The model under review builds one solid part; all positions refer to its coordinate system, in mm. A direction names the side the tool comes from. Round coordinates to 2 decimals unless told otherwise and drop trailing zeros. Loops run counter-clockwise (first coordinate to the right, second up) from the corner with the lowest first, then second, coordinate; pieces in that order, holes last. Notation, with made-up numbers: M -31,40 L -3,40 A7 cw -3,47 Z; hole C 27.25,52 d4. An arc over 180 degrees is marked long. Return JSON: item names as keys, results as strings. Group by question number.
Q1. For faces 1 (the face through (-1.825, 3.233, 1.341)), 2 (the face through (0, -2, -2)), 3 (the face through (-3, 1.5, 0)), list the 3-axis set-ups (+Z, -Z, +X, -X, +Y, -Y) from which the entire face can be reached by the end or side of a thin tool; tool diameter is ignored.
Q2. Clearance check with flat-ended pins moving along their axes: pin 1 Ø4 at (x, y) = (6, 2.5) entering from -Z; pin 2 Ø4 at (x, y) = (23, 0) entering from +Z; pin 3 Ø4 at (x, z) = (46.5, 0.5) entering from +Y. State where each tip first meets the part, or that it passes through.
Q3. To check wall thickness, follow line 1 along Y through (x, z) = (61, 1); line 2 along Z through (x, y) = (57, 0); line 3 along X through (y, z) = (2, 1). State the ranges of each line that lie inside material, in increasing order.
Q4. Draft analysis for pull direction Z (two halves, no side actions). For faces 4 (the face through (32, 0, 2)), 5 (the face through (-2.948, 0.74, -1.305)), 6 (the face through (-4, -1.3, 1.3)), 7 (the face through (-2.948, 0.761, 1.293)), state which applies: pulls with the +Z half, pulls with the -Z half, needs draft (parallel to the pull), parting line crosses it, or undercut.
Q5. Consider section A-A (x = 59.5). State the section outline as (y, z) points.
Autodesk Inventor part; units mm, degrees
ref_plane "Work Plane1" through (30, 0, 0) normal (0, -0.5, 0.866) x (1, 0, 0)
ref_plane "YZ Plane" through (0, 0, 0) normal (1, 0, 0) x (0, 1, 0)
ref_plane "XZ Plane" through (0, 0, 0) normal (0, 1, 0) x (-1, 0, 0)
sketch "Sketch1" plane through (0, 0, 0) normal (0, 0, 1) x (1, 0, 0)
  line L0 (-1, 0) -> (65, 0)
  line L1 (65, 0) -> (65, 2)
  line L2 (65, 2) -> (45, 2)
  line L3 (45, 2) -> (44.5706, 2)
  line L4 (44.5706, 2) -> (0, 2)
  line L5 (0, 2) -> (0, 3.5)
  line L6 (0, 3.5) -> (-4, 3.5)
  line L7 (-4, 3.5) -> (-4, 1.7321)
  line L8 (-4, 1.7321) -> (-2, 1.7321)
  line L9 (-2, 1.7321) -> (-1, 0)
  line L10 (-17.8, 0) -> (78.8, 0)
  line L11 (0, -0.7) -> (0, 4.2)
  line L12 (45, 2) -> (0, 2) construction
  dimension "d0" = 20
  dimension "d1" = 0.4294
  dimension "d2" = 4
  dimension "d3" = 2
  dimension "d4" = 60
  dimension "d5" = 4
  dimension "d6" = 4
  dimension "d7" = 3.4641
  dimension "d8" = 7
  dimension "d19" = 65
revolve "Body" add sketch "Sketch1" angle 360 about axis through (-1, 0, 0) along (1, 0, 0)
sketch "Sketch2" plane through (-4, 0, 0) normal (-1, 0, 0) x (0, 0, 1)
  circle A0 centre (0, 0) radius 1.7321
  line L0 (0, -4.9) -> (0, 4.9)
  line L1 (-4.9, 0) -> (4.9, 0)
  line L2 (1.7321, 0) -> (0.866, -1.5)
  line L3 (0.866, -1.5) -> (-0.866, -1.5)
  line L4 (-0.866, -1.5) -> (-1.7321, 0)
  line L5 (-1.7321, 0) -> (-0.866, 1.5)
  line L6 (-0.866, 1.5) -> (0.866, 1.5)
  line L7 (0.866, 1.5) -> (1.7321, 0)
extrude "Slot" add sketch "Sketch2" against normal up to next contours L7 A0 | A0 L2 | L6 L0 A0 | A0 L0 L3 | L0 L6 A0 | A0 L3 L0 | L4 A0 | A0 L5
fillet "Fillet2" radius 0.4 1 edges at (-4, -3.5, 0)
thread "Thread"
chamfer "Chamfer1" distance 0.4294 distance2 0.4294 1 edges at (65, -2, 0) measured on face at (65, -0.527, -0.8312)
fillet "Fillet1" radius 0.2 1 edges at (0, -2, 0)
ref_plane "Work Plane1" through (30, 0, 0) normal (0, -0.5, 0.866) x (1, 0, 0)
equation "\"d0\" = GEL"
equation "\"d1\" = GAL"
equation "\"d2\" = KOH"
equation "\"d3\" = INTI"
equation "\"d5\" = GD"
equation "\"d6\" = BDM"
equation "\"d7\" = 1.1547 * SW"
equation "\"d8\" = KOD"
equation "\"d19\" = NLG"
equation "\"d16\" = RR"
equation "\"d12\" = GEL"
equation "\"d14\" = -0.5 * SPD + 0.5 * GD"
equation "\"d15\" = GUL"
equation "\"d29\" = R"
equation "\"GD\" = NND"
equation "\"NLG\" = 65"
equation "\"GEL\" = 20"
equation "\"KOD\" = 7"
equation "\"KOH\" = 4"
equation "\"INTI\" = 2"
equation "\"GAL\" = 0.61345 * PTC"
equation "\"GUL\" = 0.61345 * PTC"
equation "\"BDM\" = NND"
equation "\"SW\" = 3"
equation "\"RR\" = 0.4"
equation "\"SPD\" = 3.14117"
equation "\"d28\" = R"
equation "\"R\" = 0.2"
equation "\"TOA\" = 30deg"
equation "\"THREADDIA\" = 4"
equation "\"KOD1\" = KOD"
equation "\"PTC\" = 0.7"
equation "\"NND\" = 4"
equation "\"E0\" = 1.155 * SW"
equation "\"GD1\" = THREADDIA - 1.2269 * PTC"
properties part number "ANSI B18.3.1M - M4x0.7 x 65, BSHCSM" material "Steel, Mild"
Values:
{
 "1": {"face 1": "+X, -X", "face 2": "+X", "face 3": "-X"},
 "2": {"pin 1": "stops at z = -1.94", "pin 2": "stops at z = 2", "pin 3": "stops at y = 2"},
 "3": {"line 1": "y = -1.73 to 1.73", "line 2": "z = -2 to 2", "line 3": "x = -4 to 0"},
 "4": {"face 4": "parting line crosses it", "face 5": "undercut", "face 6": "needs draft", "face 7": "undercut"},
 "5": {"outline": "C 0,0 d4"}
}
